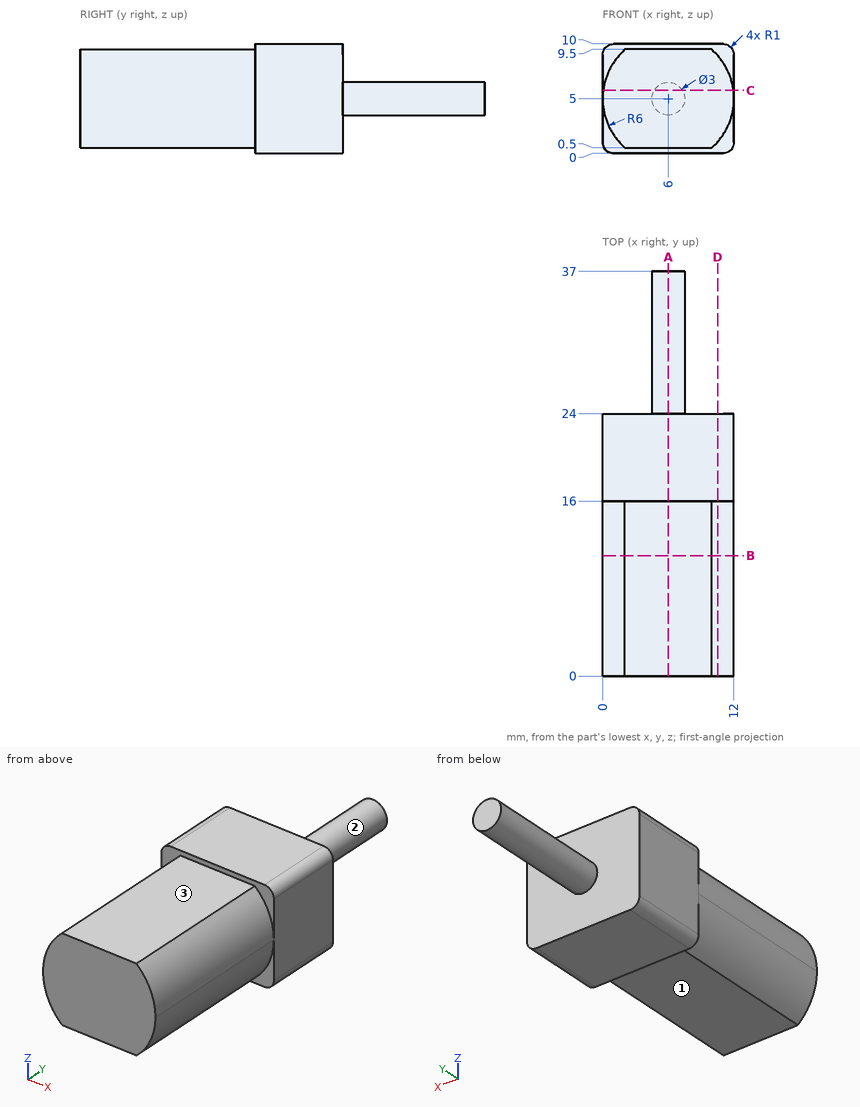
Here's the drawing with two shaded views (mm, measured from the low corner). I have some questions. A direction names the side the tool comes from. Coordinates: 2 decimals unless noted, no trailing zeros. Write each loop counter-clockwise with the first axis right and the second up, starting at its lowest first coordinate (ties: lowest second). Pieces come first, ordered by that corner, then holes. Notation, with made-up numbers: (36, 84.5) -> (91, 84.5) arc R18 cw to (91, 91.5) -> close; hole circle Ø2 at (46, 46.25). An arc over 180 degrees is marked (long way). Write item = value, one per line. Start each with the question number.
(1) I want a section at D-D (x = 10.5). Please give me the cut outline in (y, z).
(2) I want a section at B-B (y = 11). Please give me the cut outline in (x, z).
(3) Which directions (+Z, -Z, +X, -X, +Y, -Y) give clear straight access to the entire face, cutting with the end or side of a thin tool? Please do the marked faces 1, 2 and 3.
(4) I want a section at C-C (z = 5.75). Please give me the cut outline in (x, y), plus the area to 3 significant figures.
(5) I want a section at A-A (x = 6). Please give me the cut outline in (y, z).
(6) I need wall thicknesses on line 1 (Z direction, x = 4, y = 10.5); line 2 (Y direction, x = 10.5, z = 9.75); line 3 (Y direction, x = 9, z = 1.5). Which ranges of each line are inside material? Lowest first, please. Write a range as [from, to].
(7) Will these pins go through, and if not, where does the flat tip stop? pin 1 (1.5 mm diameter, centred on y = 5, z = 6, fed in from -X); pin 2 (6 mm diameter, centred on x = 3, y = 30, fed in from +Z); pin 3 (2 mm diameter, centred on x = 2, z = 4, fed in from +Y); pin 4 (1.5 mm diameter, centred on x = 2, y = 26, fed in from +Z).
Result set:
q1.outline = (0, 1.03) -> (16, 1.03) -> (16, 0) -> (24, 0) -> (24, 10) -> (16, 10) -> (16, 8.97) -> (0, 8.97) -> close
q2.outline = (2.03, 0.5) -> (9.97, 0.5) arc R6 ccw to (9.97, 9.5) -> (2.03, 9.5) arc R6 ccw to start
q3.face_1 = -Z, +X, -X, -Y
q3.face_2 = +Y
q3.face_3 = +Z, +X, -X, -Y
q4.outline = (0, 16) -> (0.05, 16) -> (0.05, 0) -> (11.95, 0) -> (11.95, 16) -> (12, 16) -> (12, 24) -> (7.3, 24) -> (7.3, 37) -> (4.7, 37) -> (4.7, 24) -> (0, 24) -> close
q4.area = 320 mm2
q5.outline = (0, 0.5) -> (16, 0.5) -> (16, 0) -> (24, 0) -> (24, 3.5) -> (37, 3.5) -> (37, 6.5) -> (24, 6.5) -> (24, 10) -> (16, 10) -> (16, 9.5) -> (0, 9.5) -> close
q6.line_1 = [0.5, 9.5]
q6.line_2 = [16, 24]
q6.line_3 = [0, 24]
q7.pin_1 = 0.01
q7.pin_2 = 6.5
q7.pin_3 = 24
q7.pin_4 = through
